CAD build for the part. Positions are in the model's coordinates, mm. Face numbers are marked on the shaded views. A direction names the side the tool comes from. Round coordinates to 2 decimals unless told otherwise and drop trailing zeros. Loops run counter-clockwise (first coordinate to the right, second up) from the corner with the lowest first, then second, coordinate; pieces in that order, holes last. Notation, with made-up numbers: (2, -21.75) - (50, -21.75) arc R33 cw to (50, 7.25) - close; hole circle Ø6 at (40, 89.25). An arc over 180 degrees is marked (long way). One line per question, with ' | ' between items.
```python
from build123d import *

# Parameters (mm, degrees)
F1_DEPTH = 63.5
F0_W     = 25.4
F0_H     = 19.05
F2_DEPTH = 25.4
F3_DEPTH = 7.9375
F5_R     = 6.35


with BuildPart() as f1:
    # F0 (on Front) → F1 (new body, symmetric)
    with BuildSketch(Plane.XZ):
        Polygon((-41.275, 9.525), (-41.275, -9.525), (41.275, -9.525), (41.275, 9.525), (22.225, 9.525), align=None)
    extrude(amount=F1_DEPTH, both=True)

    # F0 (on Front) → F2 (join, symmetric)
    with BuildSketch(Plane.XZ):
        with Locations((75.9968, 52.4002)):
            Rectangle(F0_W, F0_H)
        with BuildLine():
            Line((22.225, 9.525), (41.275, 9.525))
            Line((41.275, 9.525), (41.275, 27.0002))
            ThreePointArc((41.275, 27.0002), (45.9246798487, 38.2255201513), (57.15, 42.8752))
            Line((57.15, 42.8752), (63.2968, 42.8752))
            Line((63.2968, 42.8752), (63.2968, 61.9252))
            Line((63.2968, 61.9252), (57.15, 61.9252))
            ThreePointArc((57.15, 61.9252), (32.4542956671, 51.6959043329), (22.225, 27.0002))
            Line((22.225, 27.0002), (22.225, 9.525))
        make_face()
    extrude(amount=F2_DEPTH, both=True)

    # F0 (on Front) → F3 (join, symmetric)
    with BuildSketch(Plane.XZ):
        with BuildLine():
            add(Edge.make_bspline(
                [(-41.275, 9.525), (-32.9106339345, 31.9569138645), (12.5016221459, 71.1940555749), (57.15, 61.9252)],
                knots=[0, 0, 0, 0, 111.5045361635, 111.5045361635, 111.5045361635, 111.5045361635], degree=3))
            Line((-41.275, 9.525), (22.225, 9.525))
            Line((22.225, 9.525), (22.225, 27.0002))
            ThreePointArc((22.225, 27.0002), (32.4542956671, 51.6959043329), (57.15, 61.9252))
        make_face()
    extrude(amount=F3_DEPTH, both=True)

    # F0 (on Front) → F4 (revolve)
    with BuildSketch(Plane.XZ):
        Polygon((88.6968, 66.675), (88.6968, 61.9252), (88.6968, 42.8752), (88.6968, 38.1), (114.0968, 38.1), (114.0968, 66.675), align=None)
    revolve(axis=Axis((88.6968, 0, 52.3875), (0, 0, 1)))

    # F5
    f5_edges = [f1.edges().sort_by_distance(p)[0] for p in [
        (41.275, 63.5, 0),
        (-41.275, -63.5, 0),
        (-41.275, 63.5, 0),
        (41.275, -63.5, 0),
    ]]
    fillet(f5_edges, radius=F5_R)


solid = f1.part
```
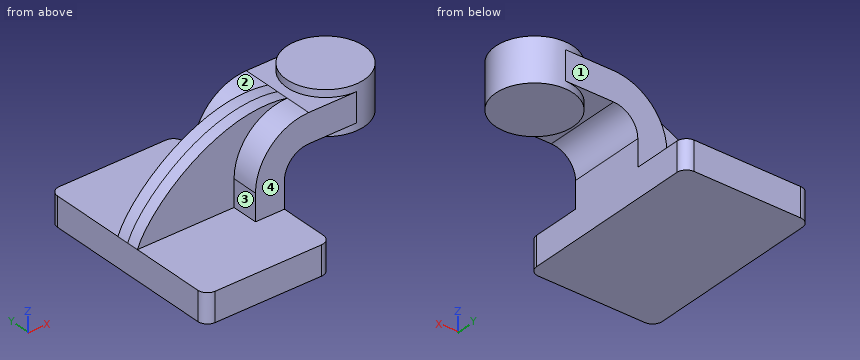
(1) Cut at D-D, the plane y = -32. Write the cut outline in (x, z) (3 decimals), then the cut area to 3 significant figures.
Results found:
outline: (-41.275, -9.525) - (41.275, -9.525) - (41.275, 9.525) - (-41.275, 9.525) - close | area: 1,570 mm²
(2) Drop flat-ended pins along their axis: P1, Ø8.5, axis at y = 14.5, z = 19, coming from the -X side (3 decimals); P2, Ø12, axis at x = 27.5, z = 31.5, coming from the +Y side; P3, Ø4, axis at x = -20, y = 30.5, coming from the +Z side (3 decimals). Give the stop position or say it passes through.
Results found:
P1: stops at x = 22.225 | P2: stops at y = 25.4 | P3: stops at z = 9.525
(3) Cut at B-B, the plane x = 83.5. Write the cut outline in (y, z) (3 decimals).
Results found:
outline: (-25.4, 42.875) - (-24.863, 42.875) - (-24.863, 38.1) - (24.863, 38.1) - (24.863, 42.875) - (25.4, 42.875) - (25.4, 61.925) - (24.863, 61.925) - (24.863, 66.675) - (-24.863, 66.675) - (-24.863, 61.925) - (-25.4, 61.925) - close
(4) Cut at A-A, the plane z = 6.5. Write the cut outline in (x, y) (3 decimals).
Results found:
outline: (-41.275, -57.15) arc R6.35 ccw to (-34.925, -63.5) - (34.925, -63.5) arc R6.35 ccw to (41.275, -57.15) - (41.275, 57.15) arc R6.35 ccw to (34.925, 63.5) - (-34.925, 63.5) arc R6.35 ccw to (-41.275, 57.15) - close
(5) Probe L1, parallel to Y at x = 3, z = 29.5; L2, parallel to Z at x = -15.5, y = -29 (3 decimals); L3, parallel to Z at x = 72, y = -14 (3 decimals). List the from-to ranges inside material, lowest first.
Results found:
L1: y = -7.94 to 7.94 | L2: z = -9.525 to 9.525 | L3: z = 38.1 to 66.675
(6) Cut at C-C, the plane y = 21. Write the cut outline in (x, z) (3 decimals), then the cut area to 3 significant figures.
Results found:
outline: (-41.275, -9.525) - (41.275, -9.525) - (41.275, 27) arc R15.875 cw to (57.15, 42.875) - (74.408, 42.875) - (74.408, 38.1) - (102.985, 38.1) - (102.985, 66.675) - (74.408, 66.675) - (74.408, 61.925) - (57.15, 61.925) arc R34.925 ccw to (22.225, 27) - (22.225, 9.525) - (-41.275, 9.525) - close | area: 3,810 mm²
(7) Tool access for the marked faces 1, 2, 3 and 4: list every direction of +Z, -Z, +X, -X, +Y, -Y with a clear straight run to the whole face (end or side of a thin tool).
Results found:
face 1: +Z, +X, -X, +Y | face 2: +Z, -X, +Y | face 3: +Z, -X, -Y | face 4: +Z, +X, -X, -Y
